```python
from build123d import *

# Parameters (mm, degrees)
BOSS_EXTRUDE2_DEPTH = 228.6
BOSS_EXTRUDE3_DEPTH = 12.7
BOSS_EXTRUDE4_DEPTH = 12.7


with BuildPart() as part:
    # Sketch5 → Boss-Extrude2 (new, symmetric)
    with BuildSketch(Plane(origin=(0, 0, 0), x_dir=(0, 0, -1), z_dir=(1, 0, 0))):
        with BuildLine():
            add(Edge.make_bspline(
                [(-28.335355673, 0), (-4.22034825, -13.482840601), (29.919203063, -7.409504984), (47.864644327, 14.230029394)],
                knots=[0, 0, 0, 0, 1, 1, 1, 1], degree=3))
            add(Edge.make_bspline(
                [(-28.335355673, 0), (-7.388023191, 23.329729693), (23.952126554, -2.21974241), (47.864644327, 14.230029394)],
                knots=[0, 0, 0, 0, 1, 1, 1, 1], degree=3))
        make_face()
    extrude(amount=BOSS_EXTRUDE2_DEPTH, both=True)

    # Sketch7 → Boss-Extrude3 (add)
    with BuildSketch(Plane(origin=(228.6, 0, 0), x_dir=(0, 0, -1), z_dir=(1, 0, 0))):
        Polygon((47.864644327, 14.230029394), (-28.530543378, 8.593586149), (-27.39909465, -16.298285859), (35.004654405, -6.81152345), (47.864644327, 7.201033869), align=None)
    extrude(amount=BOSS_EXTRUDE3_DEPTH)

    # Sketch8 → Boss-Extrude4 (add)
    with BuildSketch(Plane.ZY.offset(228.6)):
        Polygon((28.530543378, 8.593586149), (27.39909465, -16.298285859), (-35.004654405, -6.81152345), (-47.864644327, 7.201033869), (-47.864644327, 14.230029394), align=None)
    extrude(amount=BOSS_EXTRUDE4_DEPTH)


solid = part.part
```
Work out the finished part from the listing and answer in its coordinate system (mm). A direction names the side the tool comes from. Give positions to 0.01 mm unless a question says otherwise; leave off trailing zeros. Use CSV: the item, a comma, the result in double quotes. Start each with the question number.
(1) Each of these flat-tipped pins is pushed along its axis until it touches: pin 1 (1 mm diameter, centred on x = 119, y = -8, fed in from -Z); pin 2 (10 mm diameter, centred on x = 50.5, z = 4, fed in from -Y); pin 3 (3 mm diameter, centred on x = -171.5, y = 8, fed in from +Z). Where does it stop, or does it pass through?
(2) A tool of negligible diameter and unlimited length cuts with its end or side. For faces 4 (the face through (-234.861, 0.097, -41.345)), 5 (the face through (228.6, 7, 23)), 6 (the face through (-228.6, -8, -4)), from which of +Z, -Z, +X, -X, +Y, -Y can it reach the whole face along a straight path? Write none if from no direction.
(3) Find the intervals of material crossed by L1, parallel to X at y = -5.5, z = 16.5; L2, parallel to Y at x = 1.5, z = -6 (3 decimals); L3, parallel to Y at x = -63, z = -18.5, in increasing order.
(4) Determine the mould class of faces 1 (the face through (234.86, 11.45, -10.2)), 2 (the face through (-228.6, 7, 23)), 3 (the face through (-241.3, -1, -9)) for opening direction X: released by +X, released by -X, zero draft, split by the parting line, or undercut.
Results found:
1,pin 1,"through"
1,pin 2,"y = -7.14"
1,pin 3,"z = 20.28"
2,face 4,"-Z, +X, -X, -Y"
2,face 5,"+Z, +Y"
2,face 6,"-Y"
3,L1,"-241.3 to -228.6, 228.6 to 241.3"
3,L2,"-6.885 to 9.96"
3,L3,"-4.54 to 8.67"
4,face 1,"zero draft"
4,face 2,"undercut"
4,face 3,"released by -X"
